For this review, take the finished solid that the model builds, in its own axes (mm). Face numbers are marked on the shaded views. Round coordinates to 2 decimals unless told otherwise and drop trailing zeros. Order: outer loops, then holes, each group sorted by start corner. A loop starts at its lowest first (then second) coordinate and runs counter-clockwise, first axis right, second up.
Autodesk Inventor part; units mm, degrees
ref_plane "YZ Plane" through (0, 0, 0) normal (1, 0, 0) x (0, 1, 0)
ref_plane "XZ Plane" through (0, 0, 0) normal (0, 1, 0) x (-1, 0, 0)
ref_plane "XY Plane" through (0, 0, 0) normal (0, 0, 1) x (1, 0, 0)
sketch "Sketch1" plane through (0, 1.5, 0) normal (0, 0, 1) x (1, 0, 0)
  line L0 (8, 5) -> (8, -8)
  line L1 (8, -8) -> (-8, -8)
  line L2 (-8, -8) -> (-8, 5)
  line L3 (-8, 5) -> (8, 5)
  line L4 (-4.3301, 2.5) -> (-5.7735, 0)
  line L5 (-5.7735, 0) -> (-4.3301, -2.5)
  line L6 (-4.3301, -2.5) -> (-2.8868, -5)
  line L7 (-2.8868, -5) -> (0, -5)
  line L8 (0, -5) -> (2.8868, -5)
  line L9 (2.8868, -5) -> (4.3301, -2.5)
  line L10 (4.3301, -2.5) -> (5.7735, 0)
  line L11 (5.7735, 0) -> (4.3301, 2.5)
  line L12 (4.3301, 2.5) -> (2.8868, 5)
  line L13 (-2.8868, 5) -> (-4.3301, 2.5)
  point P0 (0, 0)
extrude "Extrusion1" add sketch "Sketch1" along normal blind 5 contours L0 L1 L2 L3 L13 L4 L5 L6 L7 L8 L9 L10 L11 L12
sketch "Sketch2" plane through (0, 1.5, 5) normal (0, 0, 1) x (1, 0, 0)
  line L0 (-8, 5) -> (-8, -8)
  line L1 (8, 5) -> (-8, 5)
  line L2 (8, -8) -> (8, 5)
  line L3 (-8, -8) -> (8, -8)
  circle A0 centre (0, 0) radius 3
extrude "Extrusion2" add sketch "Sketch2" along normal blind 5
properties part number "2x 2x M6 Nut Holder" material "ABS Plastic"
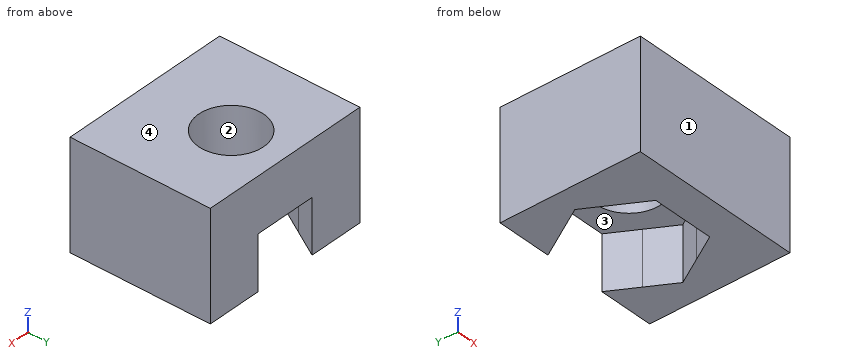
Q1. Mouldability with a two-part tool opening along Y and no side actions: class the marked faces 1, 2, 3 and 4 as +Y half, -Y half, draft (parallel to the pull), parting line (faces both ways), or undercut.
Q2. Take a section at A-A, the plane x = 0. State the section outline as (y, z) points.
Q3. Take a section at C-C, the plane z = 4.75. State the section outline as (x, y) points, plus the area to 3 significant figures.
Q4. Wall thickness on line 1 (Y direction, x = 0, z = 8.2); line 2 (X direction, y = 2.5, z = 3); line 3 (X direction, y = 0.25, z = 2.25): over which ranges is each line inside the solid? List them lowest first.
Q5. Take a section at B-B, the plane y = 2. State the section outline as (x, z) points.
Q6. Take a section at D-D, the plane y = -2.5. State the section outline as (x, z) points.
Q7. Clearance check with flat-ended pins moving along their axes: pin 1 (5 mm diameter, centred on x = -1.5, y = 1, fed in from -Z); pin 2 (5 mm diameter, centred on x = -6, y = -3.5, fed in from -Z); pin 3 (1.5 mm diameter, centred on x = 0.5, z = 3, fed in from +Y). State where each tip first meets the part, or that it passes through.
Working result:
1. face 1: -Y half
1. face 2: undercut
1. face 3: undercut
1. face 4: draft
2. outline: (-6.5, 0) - (-3.5, 0) - (-3.5, 5) - (-1.5, 5) - (-1.5, 10) - (-6.5, 10) - close; (4.5, 5) - (6.5, 5) - (6.5, 10) - (4.5, 10) - close
3. outline: (-8, -6.5) - (8, -6.5) - (8, 6.5) - (2.89, 6.5) - (4.33, 4) - (5.77, 1.5) - (4.33, -1) - (2.89, -3.5) - (-2.89, -3.5) - (-4.33, -1) - (-5.77, 1.5) - (-4.33, 4) - (-2.89, 6.5) - (-8, 6.5) - close
3. area: 121 mm2
4. line 1: y = -6.5 to -1.5, 4.5 to 6.5
4. line 2: x = -8 to -5.2, 5.2 to 8
4. line 3: x = -8 to -5.05, 5.05 to 8
5. outline: (-8, 0) - (-5.48, 0) - (-5.48, 5) - (-2.96, 5) - (-2.96, 10) - (-8, 10) - close; (2.96, 5) - (5.48, 5) - (5.48, 0) - (8, 0) - (8, 10) - (2.96, 10) - close
6. outline: (-8, 0) - (-3.46, 0) - (-3.46, 5) - (3.46, 5) - (3.46, 0) - (8, 0) - (8, 10) - (-8, 10) - close
7. pin 1: stops at z = 5
7. pin 2: stops at z = 0
7. pin 3: stops at y = -3.5
